Study the drawing (mm; zero at the part's minimum x, y, z) and answer. A direction names the side the tool comes from. Coordinates: 2 decimals unless noted, no trailing zeros. Order: outer loops, then holes, each group sorted by start corner. A loop starts at its lowest first (then second) coordinate and runs counter-clockwise, first axis right, second up.
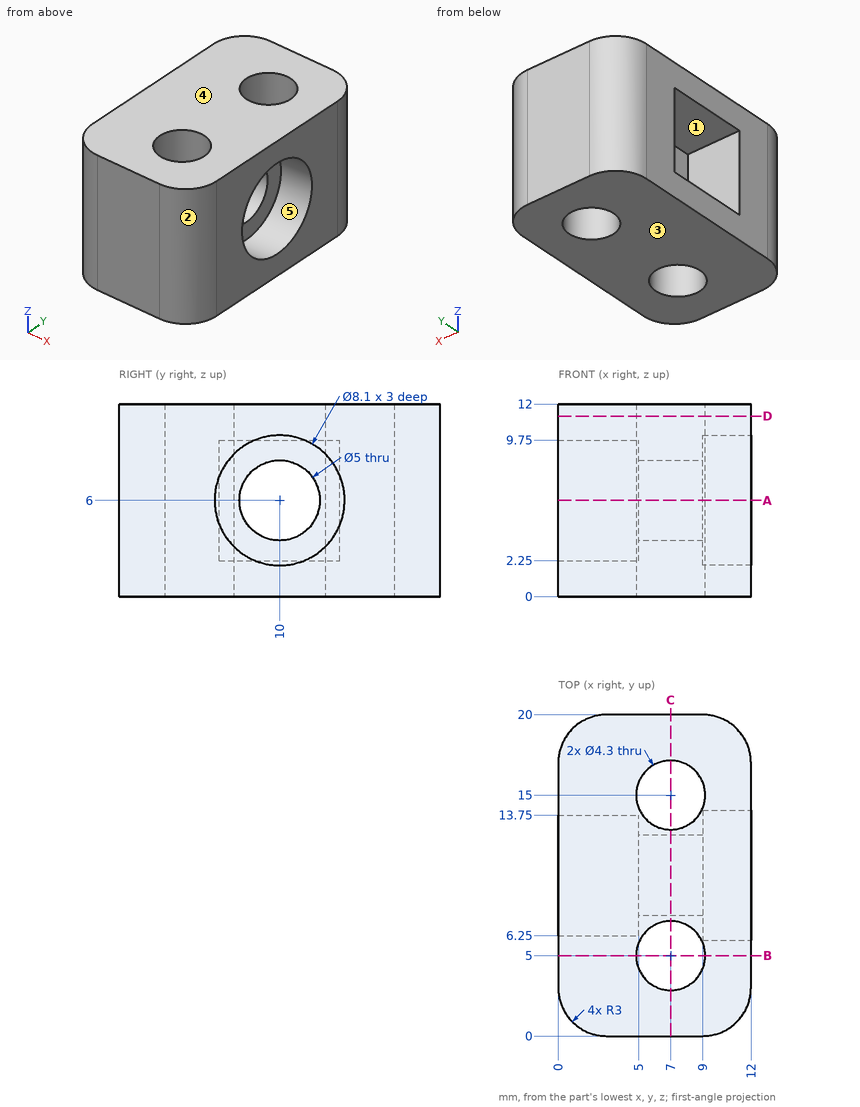
(1) Find section B-B (y = 5). Write down the section's boundary in (x, z).
(2) Consider line 1 (Y direction, x = 7, z = 6); line 2 (Y direction, x = 5.75, z = 2.25); line 3 (Y direction, x = 8.5, z = 10.75). Determine where each line is inside the solid, lowest interval first.
(3) For the marked faces 1 and 2, determine the directions among +Z, -Z, +X, -X, +Y, -Y from which every point of the face is accessible in a straight line to the end or side of a thin tool.
(4) Find section C-C (x = 7). Write down the section's boundary in (y, z).
(5) Find section D-D (z = 11.25). Write down the section's boundary in (x, y).
(6) Find section A-A (z = 6). Write down the section's boundary in (x, y), and give its area (3 significant figures).
(7) Each of these flat-tipped pins is pushed along its axis until it touches: pin 1 Ø4.5 at (y, z) = (10, 6) entering from +X; pin 2 Ø2.5 at (y, z) = (12, 6) entering from +X. Where does it stop, or does it pass through?
(8) The mould has two halves that part along Z. Classify the marked faces 3, 4 and 5: released by +Z, released by -Z, zero draft, split by the parting line, or undercut.
Findings below:
1. outline: (0, 0) - (4.85, 0) - (4.85, 12) - (0, 12) - close; (9.15, 0) - (12, 0) - (12, 12) - (9.15, 12) - close
2. line 1: y = 0 to 2.85, 7.15 to 7.5, 12.5 to 12.85, 17.15 to 20
2. line 2: y = 0 to 3.25, 6.75 to 13.25, 16.75 to 20
2. line 3: y = 0 to 3.46, 6.54 to 13.46, 16.54 to 20
3. face 1: -X
3. face 2: +Z, -Z, +X, -Y
4. outline: (0, 0) - (2.85, 0) - (2.85, 12) - (0, 12) - close; (7.15, 0) - (12.85, 0) - (12.85, 12) - (7.15, 12) - close; (17.15, 0) - (20, 0) - (20, 12) - (17.15, 12) - close; hole circle Ø5 at (10, 6)
5. outline: (0, 3) arc R3 ccw to (3, 0) - (9, 0) arc R3 ccw to (12, 3) - (12, 17) arc R3 ccw to (9, 20) - (3, 20) arc R3 ccw to (0, 17) - close; hole circle Ø4.3 at (7, 5); hole circle Ø4.3 at (7, 15)
6. outline: (0, 3) arc R3 ccw to (3, 0) - (9, 0) arc R3 ccw to (12, 3) - (12, 5.95) - (9, 5.95) - (9, 7.5) - (5, 7.5) - (5, 6.25) - (0, 6.25) - close; (0, 13.75) - (5, 13.75) - (5, 12.5) - (9, 12.5) - (9, 14.05) - (12, 14.05) - (12, 17) arc R3 ccw to (9, 20) - (3, 20) arc R3 ccw to (0, 17) - close; hole circle Ø4.3 at (7, 5); hole circle Ø4.3 at (7, 15)
6. area: 121 mm2
7. pin 1: passes through
7. pin 2: stops at x = 9
8. face 3: released by -Z
8. face 4: released by +Z
8. face 5: undercut
